```python
from build123d import *

# Parameters (mm, degrees)
F4_W     = 20
F4_H     = 25.605118
F5_DEPTH = 8
F7_DEPTH = 2.8
F8_SIZE  = 0.5


with BuildPart() as f1:
    # F0 (on Front) → F1 (revolve)
    with BuildSketch(Plane.XZ):
        Polygon((0, 8), (0, 0), (92, 0), (92, 6), (89.6, 6), (89.6, 5.5), (88.8, 5.5), (88.8, 6), (58.8, 6), (58.8, 5.5), (58, 5.5), (58, 6), (30, 6), (30, 8), align=None)
    revolve(axis=Axis((46, 0, 0), (-1, 0, 0)))

    # F4 (on offset) → F5 (cut)
    with BuildSketch(Plane.XY.offset(8)):
        with Locations((10, -2.362951)):
            Rectangle(F4_W, F4_H)
    extrude(amount=-F5_DEPTH, mode=Mode.SUBTRACT)

    # F6 (on offset) → F7 (cut)
    with BuildSketch(Plane.XY.offset(6)):
        with BuildLine():
            Line((54, 2), (34, 2))
            ThreePointArc((34, 2), (32.585786, 1.414214), (32, 0))
            ThreePointArc((32, 0), (32.585786, -1.414214), (34, -2))
            Line((34, -2), (54, -2))
            ThreePointArc((54, -2), (55.414214, -1.414214), (56, 0))
            ThreePointArc((56, 0), (55.414214, 1.414214), (54, 2))
        make_face()
    extrude(amount=-F7_DEPTH, mode=Mode.SUBTRACT)

    # F8
    f8_edges = [f1.edges().sort_by_distance(p)[0] for p in [
        (92, 0, -6),
    ]]
    chamfer(f8_edges, length=F8_SIZE)


solid = f1.part
```
Can you work these out from the model? Positions are in its coordinate system, mm. A direction names the side the tool comes from. Round coordinates to 2 decimals unless told otherwise and drop trailing zeros. Loops run counter-clockwise (first coordinate to the right, second up) from the corner with the lowest first, then second, coordinate; pieces in that order, holes last. Notation, with made-up numbers: (-32, 36.5) -> (27, 36.5) arc R23 ccw to (27, 62.5) -> close; hole circle Ø3 at (34.5, 52). An arc over 180 degrees is marked (long way). One line per item, written item: value. Start each with the question number.
1. For pin 1 (1.5 mm diameter, centred on x = 36.5, y = -1.5, fed in from +Z); pin 2 (4 mm diameter, centred on y = 0, z = 2.5, fed in from -X); pin 3 (5 mm diameter, centred on x = 78, z = 4, fed in from -Y), each with a flat end and sliding along its axis, tell me the tip position at first contact or that it passes through.
2. If we mould it in two halves opening along X, with no side actions, what happens to faces 4 (the flat face through (0, 0, -3)), 5 (the cylindrical face through (89.19, -5.37, -1.19)), 6 (the cylindrical face through (74, 0, -6)), 7 (the flat face through (30, 6, 2))? For each: pulls with the +X half, pulls with the -X half, needs draft (parallel to the pull), parting line crosses it, or undercut.
3. If we section it at B-B, the plane x = 44: Write out the boundary of the cut face in (y, z).
4. For faces 1 (the flat face through (44, -2, 4)), 2 (the flat face through (89.6, -5, 3)), 3 (the flat face through (20, 0, 3)), which set-ups out of +Z, -Z, +X, -X, +Y, -Y let a thin tool reach every point of the face, with its end or its side?
5. If I drill on probe 1 along X at (y, z) = (-2, 7.25); probe 2 along X at (y, z) = (-2.25, 0.5); probe 3 along Z at (x, y) = (12.5, 0), over which ranges is the centre line in solid material (lowest first)?
6. If we section it at A-A, the plane x = 74: Write out the boundary of the cut face in (y, z), then the cut area to 3 significant figures.
Calculated:
1. pin 1: stops at z = 5.66
1. pin 2: stops at x = 20
1. pin 3: stops at y = -5.81
2. face 4: pulls with the -X half
2. face 5: undercut
2. face 6: needs draft
2. face 7: pulls with the +X half
3. outline: (-2, 3.2) -> (-2, 5.66) arc R6 ccw (long way) to (2, 5.66) -> (2, 3.2) -> close
4. face 1: +Z
4. face 2: none
4. face 3: +Z, -X, +Y, -Y
5. probe 1: x = 20 to 30
5. probe 2: x = 20 to 92
5. probe 3: z = -8 to 0
6. outline: circle Ø12 at (0, 0)
6. area: 113 mm²
